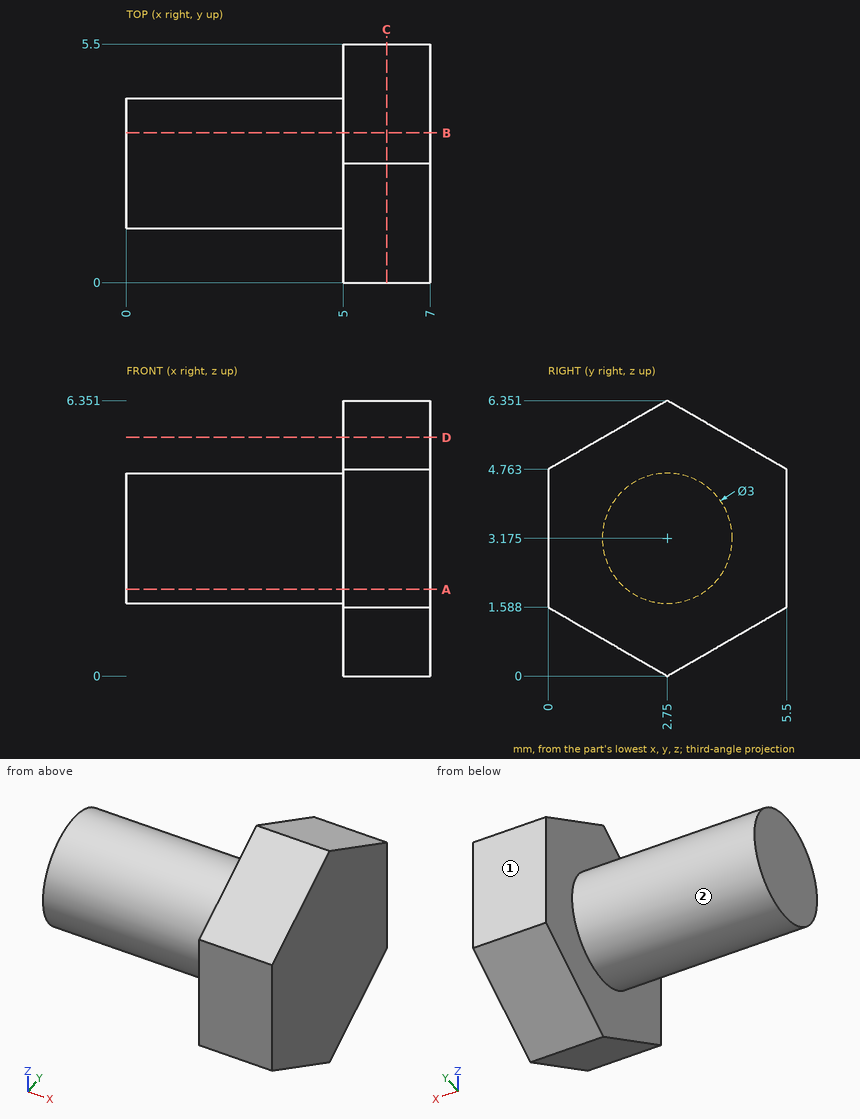
Answer from the drawing. Dimensions are ordinates in mm from the lowest x, y and z of the part. A direction names the side the tool comes from. Give positions to 0.01 mm unless a question says otherwise; leave off trailing zeros. Loops run counter-clockwise (first coordinate to the right, second up) from the corner with the lowest first, then second, coordinate; pieces in that order, holes last. Notation, with made-up numbers: (-39, -6) - (5, -6) arc R26 ccw to (5, 8) - close; hole circle Ø11 at (-15.5, -19.5). An arc over 180 degrees is marked (long way). Write each question's results on one line, items separated by ' | '.
1. Find section A-A, the plane z = 2. Write down the section's boundary in (x, y), then the cut area to 3 significant figures.
Resolved:
outline: (0, 1.82) - (5, 1.82) - (5, 0) - (7, 0) - (7, 5.5) - (5, 5.5) - (5, 3.68) - (0, 3.68) - close | area: 20.3 mm^2
2. Find section D-D, the plane z = 5.5. Write down the section's boundary in (x, y).
Resolved:
outline: (5, 1.28) - (7, 1.28) - (7, 4.22) - (5, 4.22) - close
3. Find section B-B, the plane y = 3.45. Write down the section's boundary in (x, z) (1 decimal).
Resolved:
outline: (0, 1.8) - (5, 1.8) - (5, 0.4) - (7, 0.4) - (7, 5.9) - (5, 5.9) - (5, 4.5) - (0, 4.5) - close
4. Flat-ended cylindrical pins translate along their axes: P1, Ø2, axis at y = 5, z = 4.5, coming from the -X side; P2, Ø1.5, axis at x = 1.5, y = 1, coming from the -Z side. Find the tip coordinate at first contact, or state that the pin passes through.
Resolved:
P1: stops at x = 5 | P2: stops at z = 2.06
5. Which of the six approach directions +Z, -Z, +X, -X, +Y, -Y give full straight-line access (tool end or side, diameter ignored) to the marked faces 1 and 2?
Resolved:
face 1: +Z, -Z, +X, -X, +Y | face 2: -X
6. Consider probe 1 along X at (y, z) = (1.55, 2); probe 2 along Z at (x, y) = (5.25, 1.6) (1 decimal); probe 3 along Z at (x, y) = (0.5, 1.45) (1 decimal). Determine where each line is inside the solid, lowest interval first. Write a range as from..to.
Resolved:
probe 1: x = 5..7 | probe 2: z = 0.7..5.7 | probe 3: z = 2.4..3.9
7. Find section C-C, the plane x = 6. Write down the section's boundary in (y, z).
Resolved:
outline: (0, 1.59) - (2.75, 0) - (5.5, 1.59) - (5.5, 4.76) - (2.75, 6.35) - (0, 4.76) - close
